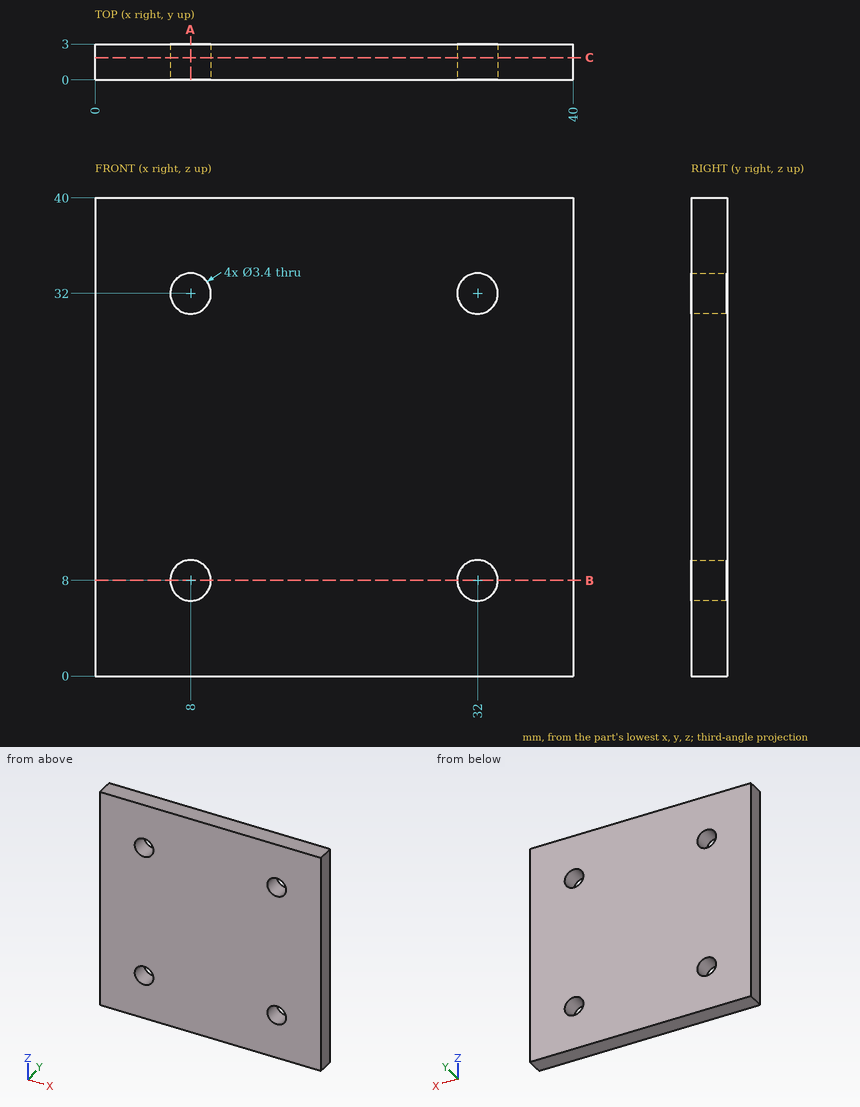
Source: three-view drawing plus pictorial views. Frame: mm from the lowest corner of the part. Round coordinates to 2 decimals unless told otherwise and drop trailing zeros. Order: outer loops, then holes, each group sorted by start corner. A loop starts at its lowest first (then second) coordinate and runs counter-clockwise, first axis right, second up. Notation, with made-up numbers: M 79.25,27.25 L 115.25,27.25 A19 cw 115.25,36.25 Z; hole C 86,-1.75 d11. An arc over 180 degrees is marked long. One line per item, written item: value.
(1) Pin query (flat end, axial travel): P1, Ø1.5, axis at x = 28, z = 20.5, coming from the -Y side. Return the tip coordinate at first contact, or that it passes through.
Result sheet:
P1: y = 0
(2) Cut plane B-B (z = 8). Return the cut outline in (x, y).
Result sheet:
outline: M 0,0 L 6.3,0 L 6.3,3 L 0,3 Z; M 9.7,0 L 30.3,0 L 30.3,3 L 9.7,3 Z; M 33.7,0 L 40,0 L 40,3 L 33.7,3 Z
(3) Cut plane A-A (x = 8). Return the cut outline in (y, z).
Result sheet:
outline: M 0,0 L 3,0 L 3,6.3 L 0,6.3 Z; M 0,9.7 L 3,9.7 L 3,30.3 L 0,30.3 Z; M 0,33.7 L 3,33.7 L 3,40 L 0,40 Z
(4) Cut plane C-C (y = 1.85). Return the cut outline in (x, z).
Result sheet:
outline: M 0,0 L 40,0 L 40,40 L 0,40 Z; hole C 8,8 d3.4; hole C 8,32 d3.4; hole C 32,8 d3.4; hole C 32,32 d3.4
(5) Line query: probe 1 along Z at (x, y) = (32, 0.4); probe 2 along X at (y, z) = (0.9, 33). Output: solid intervals per line, ascending. Write a range as [from, to].
Result sheet:
probe 1: [0, 6.3], [9.7, 30.3], [33.7, 40]
probe 2: [0, 6.63], [9.37, 30.63], [33.37, 40]
